Here's how the part is built. I have some questions about the finished solid (model axes, mm). Face numbers are marked on the shaded views. A direction names the side the tool comes from. Give positions to 0.01 mm unless a question says otherwise; leave off trailing zeros. Write each loop counter-clockwise with the first axis right and the second up, starting at its lowest first coordinate (ties: lowest second). Pieces come first, ordered by that corner, then holes. Notation, with made-up numbers: (31, 89.25) - (41, 89.25) arc R29 ccw to (41, 109.25) - close; hole circle Ø2 at (85, -29.75). An arc over 180 degrees is marked (long way). Use a Markdown table: item, result.
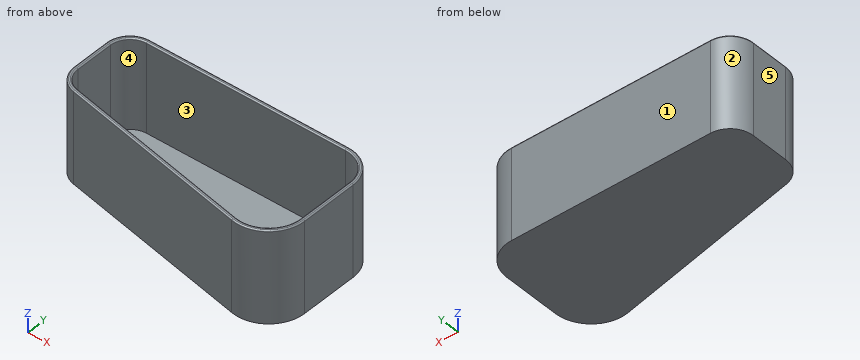
```python
from build123d import *

# Parameters (mm, degrees)
F1_DEPTH = 1
F2_DEPTH = 40
F3_R     = 0.5


with BuildPart() as f1:
    # F0 (on Top) → F1 (new body)
    with BuildSketch(Plane.XY):
        with BuildLine():
            ThreePointArc((0, -12), (-3.514719, -3.514719), (-12, 0))
            Line((-12, 0), (-98.5, 0))
            ThreePointArc((-98.5, 0), (-104.510408, -2.489592), (-107, -8.5))
            Line((-107, -8.5), (-107, -25.069857))
            ThreePointArc((-107, -25.069857), (-105.087897, -30.441041), (-100.211854, -33.395694))
            Line((-100.211854, -33.395694), (-16.819525, -50.54178))
            ThreePointArc((-16.819525, -50.54178), (-5.153344, -47.67929), (0, -36.828637))
            Line((0, -36.828637), (0, -12))
        make_face()
    extrude(amount=F1_DEPTH)

    # F0 (on Top) → F2 (join)
    with BuildSketch(Plane.XY):
        with BuildLine():
            Line((1.6, -36.828637), (1.6, -12))
            ThreePointArc((1.6, -12), (-2.383348, -2.383348), (-12, 1.6))
            Line((-12, 1.6), (-98.5, 1.6))
            ThreePointArc((-98.5, 1.6), (-105.641778, -1.358222), (-108.6, -8.5))
            Line((-108.6, -8.5), (-108.6, -25.069857))
            ThreePointArc((-108.6, -25.069857), (-106.327971, -31.452088), (-100.534086, -34.96291))
            Line((-100.534086, -34.96291), (-17.141756, -52.108996))
            ThreePointArc((-17.141756, -52.108996), (-4.142297, -48.919365), (1.6, -36.828637))
        make_face()
        with BuildLine():
            Line((-98.5, 0), (-12, 0))
            ThreePointArc((-12, 0), (-3.514719, -3.514719), (0, -12))
            Line((0, -12), (0, -36.828637))
            ThreePointArc((0, -36.828637), (-5.153344, -47.67929), (-16.819525, -50.54178))
            Line((-16.819525, -50.54178), (-100.211854, -33.395694))
            ThreePointArc((-100.211854, -33.395694), (-105.087897, -30.441041), (-107, -25.069857))
            Line((-107, -25.069857), (-107, -8.5))
            ThreePointArc((-107, -8.5), (-104.510408, -2.489592), (-98.5, 0))
        make_face(mode=Mode.SUBTRACT)
    extrude(amount=F2_DEPTH)

    # F3
    f3_edges = [f1.edges().sort_by_distance(p)[0] for p in [
        (-58.837921, -43.535953, 40),
        (-58.515689, -41.968737, 40),
    ]]
    fillet(f3_edges, radius=F3_R)


solid = f1.part
```
Item 1: Will these pins go through, and if not, where does the flat tip stop? pin 1 Ø5 at (x, z) = (-30.5, 18.5) entering from -Y; pin 2 Ø6 at (x, z) = (-67, 17.5) entering from -Y; pin 3 Ø3 at (x, z) = (-44, 28.5) entering from -Y.
Values:
| item | result |
|---|---|
| pin 1 | stops at y = -49.88 |
| pin 2 | stops at y = -42.47 |
| pin 3 | stops at y = -46.9 |
Item 2: If we section it at B-B, the plane y = -20: Write out the boundary of the cut face in (x, z), plus the area to 3 significant figures.
Values:
| item | result |
|---|---|
| outline | (-108.6, 0) - (1.6, 0) - (1.6, 39.5) arc R0.5 ccw to (1.1, 40) - (0.5, 40) arc R0.5 ccw to (0, 39.5) - (0, 1) - (-107, 1) - (-107, 39.5) arc R0.5 ccw to (-107.5, 40) - (-108.1, 40) arc R0.5 ccw to (-108.6, 39.5) - close |
| area | 235 mm2 |
Item 3: Thinking about a two-plate mould opening in X: for the marked faces 1, 2 and 3, which applies, +X half, -X half, draft (parallel to the pull), parting line (faces both ways), or undercut?
Values:
| item | result |
|---|---|
| face 1 | draft |
| face 2 | -X half |
| face 3 | undercut |
Item 4: For the marked faces 4 and 5, which set-ups out of +Z, -Z, +X, -X, +Y, -Y let a thin tool reach every point of the face, with its end or its side?
Values:
| item | result |
|---|---|
| face 4 | +Z |
| face 5 | +Z, -Z, -X, +Y, -Y |
Item 5: I need wall thicknesses on line 1 along X through (y, z) = (-21, 32.5); line 2 along Z through (x, y) = (-18.5, -38); line 3 along X through (y, z) = (-5, 9.5). Which ranges of each line are inside material? Lowest first, please. Write a range as [from, to].
Values:
| item | result |
|---|---|
| line 1 | x = [-108.6, -107], [0, 1.6] |
| line 2 | z = [0, 1] |
| line 3 | x = [-107.97, -106.25], [-2.25, -0.34] |
Item 6: If we section it at A-A, the plane z = 31.5: Write out the boundary of the cut face in (x, y), plus the area to 3 significant figures.
Values:
| item | result |
|---|---|
| outline | (-108.6, -25.07) arc R10.1 ccw to (-100.53, -34.96) - (-17.14, -52.11) arc R15.6 ccw to (1.6, -36.83) - (1.6, -12) arc R13.6 ccw to (-12, 1.6) - (-98.5, 1.6) arc R10.1 ccw to (-108.6, -8.5) - close; hole (-107, -25.07) arc R8.5 ccw to (-100.21, -33.4) - (-16.82, -50.54) arc R14 ccw to (0, -36.83) - (0, -12) arc R12 ccw to (-12, 0) - (-98.5, 0) arc R8.5 ccw to (-107, -8.5) - close |
| area | 459 mm2 |
